from build123d import *

# Parameters (mm, degrees)
F1_DEPTH = 4
F2_R     = 1.8
F4_DEPTH = 8
F3_R     = 1.8
F5_DEPTH = 8


with BuildPart() as f1:
    # F0 (on Top) → F1 (new body, symmetric)
    with BuildSketch(Plane.XY):
        with BuildLine():
            ThreePointArc((50, 5), (45.606602, 15.606602), (35, 20))
            Line((35, 20), (-35, 20))
            ThreePointArc((-35, 20), (-45.606602, 15.606602), (-50, 5))
            Line((-50, 5), (-50, -5))
            ThreePointArc((-50, -5), (-45.606602, -15.606602), (-35, -20))
            Line((-35, -20), (35, -20))
            ThreePointArc((35, -20), (45.606602, -15.606602), (50, -5))
            Line((50, -5), (50, 5))
        make_face()
    extrude(amount=F1_DEPTH, both=True)

    # F2 (on face) → F4 (cut)
    with BuildSketch(Plane(origin=(0, 0, -4), x_dir=(1, 0, 0), z_dir=(0, 0, -1))):
        with Locations((-43.311954, 5)):
            Circle(F2_R)
        with Locations((-43.436911, -5)):
            Circle(F2_R)
    extrude(amount=-F4_DEPTH, mode=Mode.SUBTRACT)

    # F3 (on face) → F5 (cut)
    with BuildSketch(Plane(origin=(0, 0, -4), x_dir=(1, 0, 0), z_dir=(0, 0, -1))):
        with Locations((44.796437, 0)):
            Circle(F3_R)
    extrude(amount=-F5_DEPTH, mode=Mode.SUBTRACT)


solid = f1.part
Design review of the part built by this model. Coordinates are the model's own, in mm. Give positions to 0.01 mm unless a question says otherwise; leave off trailing zeros. Order: outer loops, then holes, each group sorted by start corner. A loop starts at its lowest first (then second) coordinate and runs counter-clockwise, first axis right, second up.
1. To check wall thickness, follow L1, parallel to X at y = 0, z = 1; L2, parallel to X at y = 5, z = -1.75; L3, parallel to Y at x = 36.5, z = 3. State the ranges of each line that lie inside material, in increasing order.
Solution:
L1: x = -50 to 43, 46.6 to 50
L2: x = -50 to -45.24, -41.64 to 50
L3: y = -19.92 to 19.92
2. For pin 1 Ø1.5 at (y, z) = (-11, -2) entering from +X; pin 2 Ø4 at (y, z) = (-8.5, -2) entering from -X, all flat-tipped, find the tip position at first contact; note any pin that passes through.
Solution:
pin 1: stops at x = 49.05
pin 2: stops at x = -49.92
3. Add section B-B, the plane z = 0.5. State the section outline as (x, y) points, then the cut area to 3 significant figures.
Solution:
outline: (-50, -5) arc R15 ccw to (-35, -20) - (35, -20) arc R15 ccw to (50, -5) - (50, 5) arc R15 ccw to (35, 20) - (-35, 20) arc R15 ccw to (-50, 5) - close; hole circle Ø3.6 at (-43.44, 5); hole circle Ø3.6 at (-43.31, -5); hole circle Ø3.6 at (44.8, 0)
area: 3,780 mm2
4. Add section C-C, the plane y = -12.5. State the section outline as (x, z) points, then the cut area to 3 significant figures.
Solution:
outline: (-47.99, -4) - (47.99, -4) - (47.99, 4) - (-47.99, 4) - close
area: 768 mm2
5. Add section A-A, the plane y = 0. State the section outline as (x, z) points.
Solution:
outline: (-50, -4) - (43, -4) - (43, 4) - (-50, 4) - close; (46.6, -4) - (50, -4) - (50, 4) - (46.6, 4) - close
